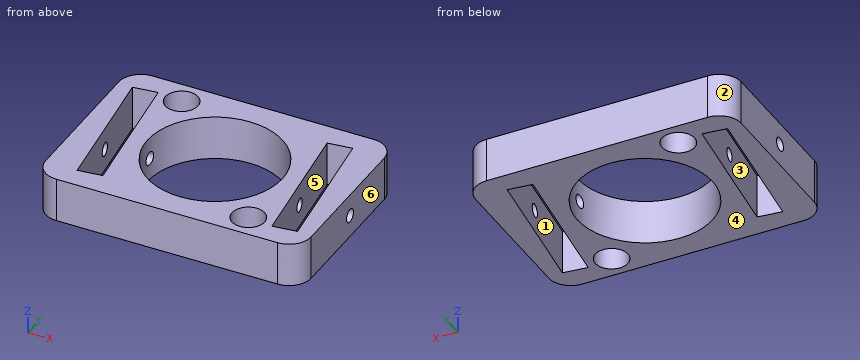
```python
from build123d import *

# Parameters (mm, degrees)
F0_R     = 3.7
F0_R_2   = 15.25
F1_DEPTH = 10
F2_R     = 1.5
F3_DEPTH = 12.5
F4_R     = 1.5
F5_DEPTH = 12.5


with BuildPart() as f1:
    # F0 (on Top) → F1 (new body)
    with BuildSketch(Plane.XY):
        with BuildLine():
            Line((25, 21), (0, 21))
            Line((0, 21), (-25, 21))
            ThreePointArc((-25, 21), (-28.5355339059, 19.5355339059), (-30, 16))
            Line((-30, 16), (-30, 0))
            Line((-30, 0), (-30, -16))
            ThreePointArc((-30, -16), (-28.5355339059, -19.5355339059), (-25, -21))
            Line((-25, -21), (0, -21))
            Line((0, -21), (25, -21))
            ThreePointArc((25, -21), (28.5355339059, -19.5355339059), (30, -16))
            Line((30, -16), (30, 0))
            Line((30, 0), (30, 16))
            ThreePointArc((30, 16), (28.5355339059, 19.5355339059), (25, 21))
        make_face()
        with Locations((15.5563491861, -15.5563491861)):
            Circle(F0_R, mode=Mode.SUBTRACT)
        Polygon((22.7795924225, 16.2158791206), (24.729501917, 0.3351406944), (26.6794114115, -15.5455977319), (21.2204075775, -16.2158791206), (17.3205885885, 15.5455977319), align=None, mode=Mode.SUBTRACT)
        Polygon((-21.2204075775, 16.2158791206), (-19.270498083, 0.3351406944), (-17.3205885885, -15.5455977319), (-22.7795924225, -16.2158791206), (-24.729501917, -0.3351406944), (-26.6794114115, 15.5455977319), align=None, mode=Mode.SUBTRACT)
        with Locations((-15.5563491861, 15.5563491861)):
            Circle(F0_R, mode=Mode.SUBTRACT)
        Circle(F0_R_2, mode=Mode.SUBTRACT)
    extrude(amount=F1_DEPTH)

    # F2 (on face) → F3 (cut, symmetric)
    with BuildSketch(Plane(origin=(-18.943751072, -2.3260001572, 0), x_dir=(0.1218693434, -0.9925461516, 0), z_dir=(-0.9925461516, -0.1218693434, 0))):
        with Locations((-2.6811255549, 5)):
            Circle(F2_R)
    extrude(amount=F3_DEPTH, both=True, mode=Mode.SUBTRACT)

    # F4 (on face) → F5 (cut, symmetric)
    with BuildSketch(Plane(origin=(18.943751072, 2.3260001572, 0), x_dir=(-0.1218693434, 0.9925461516, 0), z_dir=(0.9925461516, 0.1218693434, 0))):
        with Locations((-2.6811255549, 5)):
            Circle(F4_R)
    extrude(amount=F5_DEPTH, both=True, mode=Mode.SUBTRACT)


solid = f1.part
```
Input: part model. Units: mm. Frame: model coordinates. Face numbers are marked on the shaded views. A direction names the side the tool comes from. Coordinates: 2 decimals unless noted, no trailing zeros. Loops run counter-clockwise (first coordinate to the right, second up) from the corner with the lowest first, then second, coordinate; pieces in that order, holes last. Notation, with made-up numbers: M 34.5,29.5 L 91.5,29.5 A19 ccw 91.5,62.5 Z; hole C 41.25,-24 d8. An arc over 180 degrees is marked long. One line per item, written item: value.
(1) Section B-B (z = 7.25). Output: boundary loops of the cut face in (x, y), and give its area (3 significant figures).
Filled in:
outline: M -30,-16 A5 ccw -25,-21 L 25,-21 A5 ccw 30,-16 L 30,16 A5 ccw 25,21 L -25,21 A5 ccw -30,16 Z; hole M -26.68,15.55 L -22.78,-16.22 L -17.32,-15.55 L -21.22,16.22 Z; hole C -15.56,15.56 d7.4; hole C 0,0 d30.5; hole C 15.56,-15.56 d7.4; hole M 17.32,15.55 L 21.22,-16.22 L 26.68,-15.55 L 22.78,16.22 Z
area: 1,330 mm^2
(2) Section C-C (y = -14.5). Output: boundary loops of the cut face in (x, z).
Filled in:
outline: M -30,0 L -22.99,0 L -22.99,10 L -30,10 Z; M -17.45,0 L -4.72,0 L -4.72,10 L -17.45,10 Z; M 4.72,0 L 12.01,0 L 12.01,10 L 4.72,10 Z; M 19.1,0 L 21.01,0 L 21.01,10 L 19.1,10 Z; M 26.55,0 L 30,0 L 30,10 L 26.55,10 Z
(3) Line query: line 1 along Y through (x, z) = (0, 4); line 2 along X through (y, z) = (-11, 9.5); line 3 along X through (y, z) = (-15.5, 1). Output: solid intervals per line, ascending. Write a range as from..to.
Filled in:
line 1: -21..-15.25, 15.25..21
line 2: -30..-23.42, -17.88..-10.56, 10.56..20.58, 26.12..30
line 3: -30..-22.87, -17.33..11.86, 19.26..21.13, 26.67..30
(4) Pull-direction query (X, two-part tool) for the marked faces 3, 4, 5 and 6; classes: +X half, -X half, draft (parallel to the pull), parting line (faces both ways), or undercut.
Filled in:
face 3: undercut
face 4: draft
face 5: undercut
face 6: +X half
(5) Reachability of the marked faces 1 and 2 from +Z, -Z, +X, -X, +Y, -Y: full face, straight path, thin tool, end or side. Return the list, or none.
Filled in:
face 1: +Z, -Z
face 2: +Z, -Z, -X, +Y
(6) Pin query (flat end, axial travel): pin 1 (12 mm diameter, centred on x = -15.56, y = 15.56, fed in from -Z). Return the tip coordinate at first contact, or that it passes through.
Filled in:
pin 1: z = 0
(7) Section D-D (y = 7). Output: boundary loops of the cut face in (x, z).
Filled in:
outline: M -30,0 L -25.63,0 L -25.63,10 L -30,10 Z; M -20.09,0 L -13.55,0 L -13.55,10 L -20.09,10 Z; M 13.55,0 L 18.37,0 L 18.37,10 L 13.55,10 Z; M 23.91,0 L 30,0 L 30,10 L 23.91,10 Z
(8) Section A-A (x = 0). Output: boundary loops of the cut face in (y, z), and give its area (3 significant figures).
Filled in:
outline: M -21,0 L -15.25,0 L -15.25,10 L -21,10 Z; M 15.25,0 L 21,0 L 21,10 L 15.25,10 Z
area: 115 mm^2
